```python
from build123d import *

# Parameters (mm, degrees)
SKETCH1_W            = 152.4
SKETCH1_H            = 76.2
BOSS_EXTRUDE1_DEPTH  = 3.175
SKETCH2_R            = 1.545336663
CUT_EXTRUDE4_DEPTH   = 86.253332046
SKETCH3_W            = 134.7
SKETCH3_H            = 3.175
BOSS_EXTRUDE2_DEPTH  = 3.175
CUT_SWEEP1_PROFILE_R = 12.7


with BuildPart() as part:
    # Sketch1 → Boss-Extrude1 (new body)
    with BuildSketch(Plane(origin=(0, 0, 0), x_dir=(1, 0, 0), z_dir=(0, 1, 0))):
        Rectangle(SKETCH1_W, SKETCH1_H)
    extrude(amount=BOSS_EXTRUDE1_DEPTH)

    # Sketch2 → Cut-Extrude4 (cut, through all)
    with BuildSketch(Plane(origin=(0, 3.175, 0), x_dir=(1, 0, 0), z_dir=(0, 1, 0))):
        Polygon((-58.5, 12.6), (-58.5, -38.1), (76.2, -38.1), (76.2, 38.1), (58.5, 38.1), (58.5, 12.6), (56.5, 12.6), (41.5, 26.6), (41.5, 32.45), (-41.5, 32.45), (-41.5, 26.6), (-56.5, 12.6), align=None)
        with Locations(Location((-52.505245516, 25.605245516, 0), (0, 0, 270))):
            Circle(SKETCH2_R)
        with Locations(Location((52.5, 25.605245516, 0), (0, 0, 270))):
            Circle(SKETCH2_R)
    extrude(amount=-CUT_EXTRUDE4_DEPTH, mode=Mode.SUBTRACT)

    # Sketch3 → Boss-Extrude2 (add)
    with BuildSketch(Plane(origin=(0, 0, -38.1), x_dir=(-1, 0, 0), z_dir=(0, 0, -1))):
        with Locations((8.85, 1.5875)):
            Rectangle(SKETCH3_W, SKETCH3_H)
    extrude(amount=BOSS_EXTRUDE2_DEPTH)

    # Cut-Sweep1: sweep along a curve in space
    with BuildLine() as cut_sweep1_path:
        Line((-83.9, 3.175, 467.883912637), (-83.9, 3.175, -36.654630794))
        Line((-83.9, 3.175, -36.654630794), (-83.9, 3.175, -210.183283037))
    # Cut-Sweep1 profile (on start of the path) → Cut-Sweep1 (sweep, cut)
    with BuildSketch(Plane(origin=(-83.9, 3.175, 467.883912637), x_dir=(-1, 0, 0), z_dir=(0, 0, -1))):
        Circle(CUT_SWEEP1_PROFILE_R)
    sweep(path=cut_sweep1_path.line, mode=Mode.SUBTRACT)


solid = part.part
```
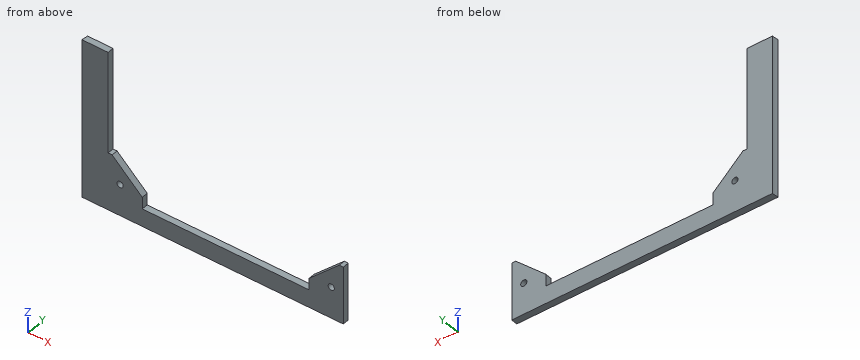
Could you check a few things on this model? Use its own coordinates, in mm. Give positions to 0.01 mm unless a question says otherwise; leave off trailing zeros. Order: outer loops, then holes, each group sorted by start corner. A loop starts at its lowest first (then second) coordinate and runs counter-clockwise, first axis right, second up.
Q1. If I drill on line 1 along X through (y, z) = (2.9, -29); line 2 along X through (y, z) = (2.85, -19.5); line 3 along X through (y, z) = (2.9, -36), over which ranges is the centre line in solid material (lowest first)?
Q2. Suppose I cut it at D-D, the plane x = -32.5. Write out the boundary of the cut face in (y, z) (3 decimals).
Q3. Suppose I cut it at B-B, the plane x = 52.5. Write out the boundary of the cut face in (y, z) (3 decimals).
Q4. Suppose I cut it at C-C, the plane z = 29. Write out the boundary of the cut face in (x, y) (3 decimals).
Q5. I'm going to push flat-ended pins straight in: P1, Ø1, axis at x = -18, y = 1, coming from the +Z side; P2, Ø0.6, axis at x = -58, y = 1.5, coming from the +Z side. Where does each tip first touch, or does it pass through?
Q6. Suppose I cut it at A-A, the plane y = 0.8. Write out the boundary of the cut face in (x, z) (3 decimals).
Solution:
1. line 1: x = -71.2 to -41.5, 41.5 to 58.5
1. line 2: x = -71.2 to -49.11, 49.11 to 58.5
1. line 3: x = -71.2 to 58.5
2. outline: (0, -41.275) - (3.175, -41.275) - (3.175, -32.45) - (0, -32.45) - close
3. outline: (0, -41.275) - (3.175, -41.275) - (3.175, -27.151) - (0, -27.151) - close; (0, -24.06) - (3.175, -24.06) - (3.175, -16.333) - (0, -16.333) - close
4. outline: (-71.603, 0) - (-58.5, 0) - (-58.5, 3.175) - (-71.2, 3.175) arc R12.7 cw to start
5. P1: stops at z = -32.45
5. P2: stops at z = -12.6
6. outline: (-71.424, -41.275) - (58.5, -41.275) - (58.5, -12.6) - (56.5, -12.6) - (41.5, -26.6) - (41.5, -32.45) - (-41.5, -32.45) - (-41.5, -26.6) - (-56.5, -12.6) - (-58.5, -12.6) - (-58.5, 38.1) - (-71.424, 38.1) - close; hole circle Ø3.091 at (-52.505, -25.605); hole circle Ø3.091 at (52.5, -25.605)
